```python
from build123d import *

# Parameters (mm, degrees)
BOSS_EXTRUDE1_START     = 7.6
SKETCH1_R               = 4
BOSS_EXTRUDE1_DEPTH     = 2
BOSS_EXTRUDE2_START     = -7.6
SKETCH1_2_R             = 4
BOSS_EXTRUDE2_DEPTH     = 2
BOSS_EXTRUDE3_START     = -7.6
SKETCH2_W               = 2
SKETCH2_H               = 20
BOSS_EXTRUDE3_DEPTH     = 15.2
SKETCH3_R               = 12.7
CUT_EXTRUDE1_DEPTH      = 13
CUT_EXTRUDE1_DEPTH_BACK = 13


with BuildPart() as part:
    # Sketch1 → Boss-Extrude1 (new body)
    with BuildSketch(Plane(origin=(0, 0, 0), x_dir=(1, 0, 0), z_dir=(0, 1, 0)).offset(BOSS_EXTRUDE1_START)):
        with BuildLine():
            Line((7.06, 27.5), (12, 27.5))
            Line((12, 27.5), (12, 7.5))
            Line((12, 7.5), (7.332619485, -3.198857842))
            ThreePointArc((7.332619485, -3.198857842), (0, -8), (-7.332619485, -3.198857842))
            Line((-7.332619485, -3.198857842), (-12, 7.5))
            Line((-12, 7.5), (-12, 22.888900714))
            Line((-12, 22.888900714), (-12, 27.5))
            Line((-12, 27.5), (7.06, 27.5))
        make_face()
        Circle(SKETCH1_R, mode=Mode.SUBTRACT)
    extrude(amount=BOSS_EXTRUDE1_DEPTH)



with BuildPart() as body_2:
    # Sketch1<2> → Boss-Extrude2 (new body)
    with BuildSketch(Plane(origin=(0, 0, 0), x_dir=(1, 0, 0), z_dir=(0, 1, 0)).offset(BOSS_EXTRUDE2_START)):
        with BuildLine():
            Line((7.06, 27.5), (12, 27.5))
            Line((12, 27.5), (12, 7.5))
            Line((12, 7.5), (7.332619485, -3.198857842))
            ThreePointArc((7.332619485, -3.198857842), (0, -8), (-7.332619485, -3.198857842))
            Line((-7.332619485, -3.198857842), (-12, 7.5))
            Line((-12, 7.5), (-12, 22.888900714))
            Line((-12, 22.888900714), (-12, 27.5))
            Line((-12, 27.5), (7.06, 27.5))
        make_face()
        Circle(SKETCH1_2_R, mode=Mode.SUBTRACT)
    extrude(amount=-BOSS_EXTRUDE2_DEPTH)


with BuildPart() as part_1:
    add(part.part)

    add(body_2.part)  # Boss-Extrude3 merges body 2
    # Sketch2 → Boss-Extrude3 (add)
    with BuildSketch(Plane(origin=(0, 0, 0), x_dir=(1, 0, 0), z_dir=(0, 1, 0)).offset(BOSS_EXTRUDE3_START)):
        with Locations((-11, 17.5)):
            Rectangle(SKETCH2_W, SKETCH2_H)
        with Locations((11, 17.5)):
            Rectangle(SKETCH2_W, SKETCH2_H)
    extrude(amount=BOSS_EXTRUDE3_DEPTH)

    # Sketch3 → Cut-Extrude1 (cut, two sides)
    with BuildSketch(Plane(origin=(0, 0, 0), x_dir=(0, 0, -1), z_dir=(1, 0, 0))) as cut_extrude1_sk:
        with Locations((37.4, 0)):
            Circle(SKETCH3_R)
    extrude(amount=CUT_EXTRUDE1_DEPTH, mode=Mode.SUBTRACT)
    extrude(cut_extrude1_sk.sketch, amount=-CUT_EXTRUDE1_DEPTH_BACK, mode=Mode.SUBTRACT)


solid = part_1.part
```
Could you check a few things on this model? Use its own coordinates, in mm. A direction names the side the tool comes from. Give positions to 0.01 mm unless a question says otherwise; leave off trailing zeros. Write each loop counter-clockwise with the first axis right and the second up, starting at its lowest first coordinate (ties: lowest second). Pieces come first, ordered by that corner, then holes. Notation, with made-up numbers: (-23.5, 73.25) - (-13.5, 73.25) arc R12 cw to (-13.5, 77.25) - close; hole circle Ø5 at (25, 22). An arc over 180 degrees is marked (long way). One line per item, written item: value. Start each with the question number.
Item 1: Imagine slicing it at B-B, the plane y = -5.25. List the corners of the cut face in (x, z) for me, and give its area (3 significant figures).
Item 2: Please list where these lines run through material, in increasing order: line 1 (Z direction, x = 0, y = -8.8); line 2 (Y direction, x = -2, z = -14); line 3 (X direction, y = -3.75, z = -14). Write a range as from..to.
Item 3: Which directions (+Z, -Z, +X, -X, +Y, -Y) give clear straight access to the entire face, cutting with the end or side of a thin tool? Please do faces 1 (the face through (-10, 0, -17)), 2 (the face through (11, 0, -7.5)), 3 (the face through (12, 0, -18)).
Item 4: Imagine slicing it at D-D, the plane x = 0. List the corners of the cut face in (y, z) for me, and give its area (3 significant figures).
Item 5: Imagine slicing it at C-C, the plane z = 0. List the corners of the cut face in (x, y) for me, and give its area (3 significant figures).
Item 6: If we mould it in two halves opening along Z, with no side actions, what happens to faces 4 (the face through (-0.867, -8.586, 3.905)), 5 (the face through (9.7, 8.59, -2.23)), 6 (the face through (-0.867, 8.586, 3.905)), 7 (the face through (0, 9.6, -14))? For each: +Z half, -Z half, draft (parallel to the pull), parting line (faces both ways), or undercut.
Item 7: I'm going to push flat-ended pins straight in: pin 1 (1 mm diameter, centred on x = -10.5, y = -1.5, fed in from +Z); pin 2 (5 mm diameter, centred on x = -4.5, y = -3.5, fed in from +Z). Where does each tip first touch, or does it pass through?
Item 8: Imagine slicing it at A-A, the plane x = -6. List the corners of the cut face in (y, z) for me.
Geometry says:
1. outline: (-12, -25.84) - (-10, -25.84) - (-10, -7.5) - (-12, -7.5) - close; (10, -25.84) - (12, -25.84) - (12, -7.5) - (10, -7.5) - close
1. area: 73.3 mm^2
2. line 1: -27.5..-4, 4..8
2. line 2: -9.6..-7.6, 7.6..9.6
2. line 3: -12..-10, 10..12
3. face 1: +Z, -Z
3. face 2: +Z, +X, -X
3. face 3: +Z, -Z, +X, +Y, -Y
4. outline: (-9.6, -27.5) - (-7.95, -27.5) arc R12.7 cw to (-7.6, -27.23) - (-7.6, -4) - (-9.6, -4) - close; (-9.6, 4) - (-7.6, 4) - (-7.6, 8) - (-9.6, 8) - close; (7.6, -27.23) arc R12.7 cw to (7.95, -27.5) - (9.6, -27.5) - (9.6, -4) - (7.6, -4) - close; (7.6, 4) - (9.6, 4) - (9.6, 8) - (7.6, 8) - close
4. area: 110 mm^2
5. outline: (-8.73, -9.6) - (-4, -9.6) - (-4, -7.6) - (-8.73, -7.6) - close; (-8.73, 7.6) - (-4, 7.6) - (-4, 9.6) - (-8.73, 9.6) - close; (4, -9.6) - (8.73, -9.6) - (8.73, -7.6) - (4, -7.6) - close; (4, 7.6) - (8.73, 7.6) - (8.73, 9.6) - (4, 9.6) - close
5. area: 37.8 mm^2
6. face 4: undercut
6. face 5: +Z half
6. face 6: undercut
6. face 7: draft
7. pin 1: z = -7.5
7. pin 2: through
8. outline: (-9.6, -27.5) - (-7.95, -27.5) arc R12.7 cw to (-7.6, -27.23) - (-7.6, 5.29) - (-9.6, 5.29) - close; (7.6, -27.23) arc R12.7 cw to (7.95, -27.5) - (9.6, -27.5) - (9.6, 5.29) - (7.6, 5.29) - close
